Here's how the part is built. I have some questions about the finished solid (model axes, mm). Face numbers are marked on the shaded views. A direction names the side the tool comes from. Round coordinates to 2 decimals unless told otherwise and drop trailing zeros. Write each loop counter-clockwise with the first axis right and the second up, starting at its lowest first coordinate (ties: lowest second). Pieces come first, ordered by that corner, then holes. Notation, with made-up numbers: M 59.25,-11 L 83.25,-11 A15 ccw 83.25,10 Z; hole C 71.5,15 d4. An arc over 180 degrees is marked long. Use one line per item in the form item = value. Start each with the question number.
Q1. I want a section at A-A on y = -73. List the corners of the cut face in (x, z) for me, and give its area (3 significant figures).
Q2. For the marked faces 1, 2 and 3, which set-ups out of +Z, -Z, +X, -X, +Y, -Y let a thin tool reach every point of the face, with its end or its side?
Q3. I need wall thicknesses on line 1 along Z through (x, y) = (-0.25, -24); line 2 along Y through (x, z) = (3.5, 1). Which ranges of each line are inside material? Lowest first, please. Write a range as from..to.
Q4. I'm going to push flat-ended pins straight in: pin 1 Ø1 at (x, y) = (2.5, -22) entering from +Z; pin 2 Ø2 at (y, z) = (-34, 2.5) entering from -X; pin 3 Ø1.5 at (y, z) = (-16.5, 2.5) entering from +X; pin 4 Ø2.5 at (x, z) = (-1, 0) entering from +Y. Where does each tip first touch, or does it pass through?
```python
from build123d import *

# Parameters (mm, degrees)
SKETCH1_W           = 4.5
SKETCH1_H           = 68
SKETCH2_R           = 3.25
BOSS_EXTRUDE1_DEPTH = 5
BOSS_EXTRUDE2_START = 7
SKETCH3_R           = 3.25
BOSS_EXTRUDE2_DEPTH = 7
CHAMFER1_SIZE       = 1.5
CHAMFER1_SIZE2      = 0.866025404
SKETCH4_R           = 2.383974596
BOSS_EXTRUDE3_DEPTH = 1.23
FILLET1_R           = 3


with BuildPart() as part:
    # Sketch1 → Revolve1 (revolve)
    with BuildSketch(Plane.XY, mode=Mode.PRIVATE) as revolve1_sk:
        with Locations((-2.25, 0)):
            Rectangle(SKETCH1_W, SKETCH1_H)
    revolve(revolve1_sk.sketch.rotate(Axis((0, 43.52476671, 0), (0, -1, 0)), 270), axis=Axis((0, 43.52476671, 0), (0, -1, 0)))

    # Sketch2 → Boss-Extrude1 (add)
    with BuildSketch(Plane.XZ.offset(34)):
        with Locations(Location((0, 0, 0), (0, 0, 270))):
            Circle(SKETCH2_R)
    extrude(amount=BOSS_EXTRUDE1_DEPTH)

    # Sketch3 → Boss-Extrude2 (add)
    with BuildSketch(Plane(origin=(0, 34, 0), x_dir=(1, 0, 0), z_dir=(0, 1, 0)).offset(BOSS_EXTRUDE2_START)):
        with Locations(Location((0, 0, 0), (0, 0, 90))):
            Circle(SKETCH3_R)
    extrude(amount=-BOSS_EXTRUDE2_DEPTH)

    # Chamfer1
    chamfer1_edges = [part.edges().sort_by_distance(p)[0] for p in [
        (0, 41, 3.25),
    ]]
    chamfer1_side = [part.faces().sort_by_distance(p)[0] for p in [
        (0, 37.5, 3.25),
    ]]
    chamfer(chamfer1_edges, length=CHAMFER1_SIZE, length2=CHAMFER1_SIZE2, reference=chamfer1_side[0])

    # Sketch4 → Boss-Extrude3 (add)
    with BuildSketch(Plane(origin=(0, 41, 0), x_dir=(1, 0, 0), z_dir=(0, 1, 0))):
        with Locations(Location((0, 0, 0), (0, 0, 270))):
            Circle(SKETCH4_R)
    extrude(amount=BOSS_EXTRUDE3_DEPTH)

    # Sketch5 → Revolve2 (revolve)
    with BuildSketch(Plane(origin=(0, 0, 0), x_dir=(0, 0, -1), z_dir=(1, 0, 0))):
        Polygon((0, 47.23), (-2, 45.23), (-2, 42.23), (0, 42.23), align=None)
    revolve(axis=Axis((0, 53.154384726, 0), (0, -1, 0)))

    # Fillet1
    fillet1_edges = [part.edges().sort_by_distance(p)[0] for p in [
        (0, 45.23, -2),
    ]]
    fillet(fillet1_edges, radius=FILLET1_R)


with BuildPart() as part_1:
    # Body-Move/Copy1: moved
    add(part.part.moved(Location((0, -47.23, 0))))


solid = part_1.part
```
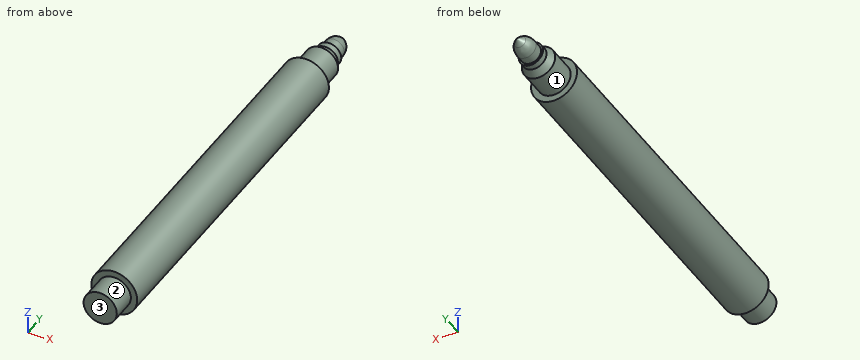
Reported:
q1.outline = C 0,0 d9
q1.area = 63.6 mm^2
q2.face_1 = +Y
q2.face_2 = -Y
q2.face_3 = +Z, -Z, +X, -X, -Y
q3.line_1 = -4.49..4.49
q3.line_2 = -81.23..-13.23
q4.pin_1 = 4.03
q4.pin_2 = -4.24
q4.pin_3 = 4.15
q4.pin_4 = 0
